```python
from build123d import *

# Parameters (mm, degrees)
F1_DEPTH = 4.6
F2_R     = 1.05
F3_DEPTH = 25


with BuildPart() as f1:
    # F0 (on Top) → F1 (new body)
    with BuildSketch(Plane.XY):
        Polygon((-15.24, 0), (0, 0), (0, 19.245), (-15.24, 19.245), (-15.24, 16.245), (-3, 16.245), (-3, 3), (-15.24, 3), align=None)
    extrude(amount=F1_DEPTH)

    # F2 (on face) → F3 (cut)
    with BuildSketch(Plane.XZ):
        with Locations((-7.62, 2.3)):
            Circle(F2_R)
    extrude(amount=-F3_DEPTH, mode=Mode.SUBTRACT)


solid = f1.part
```
Verification items for the finished model (mm, model axes). A direction names the side the tool comes from. Coordinates: 2 decimals unless noted, no trailing zeros. Loops run counter-clockwise (first coordinate to the right, second up) from the corner with the lowest first, then second, coordinate; pieces in that order, holes last. Notation, with made-up numbers: (80.5, -32) - (126.5, -32) arc R17 ccw to (126.5, -4) - close; hole circle Ø1 at (42.5, -35.75). An arc over 180 degrees is marked (long way). Return JSON: item names as keys, results as strings.
1. Section check C-C, the plane x = -7.62. Record the boundary of the cut face in (y, z) (3 decimals), then the cut area to 3 significant figures.
Established:
{"outline": "(0, 0) - (3, 0) - (3, 1.25) - (0, 1.25) - close; (0, 3.35) - (3, 3.35) - (3, 4.6) - (0, 4.6) - close; (16.245, 0) - (19.245, 0) - (19.245, 1.25) - (16.245, 1.25) - close; (16.245, 3.35) - (19.245, 3.35) - (19.245, 4.6) - (16.245, 4.6) - close", "area": "15.0 mm2"}
2. Mould release check, pull along X, two halves, no side actions. Record for faces 1 (the cylindrical face through (-8.45, 17.72, 1.66)), 2 (the flat face through (-15.24, 18, 2)), 3 (the flat face through (-2.6, 9.8, 0)): +X half, -X half, draft (parallel to the pull), parting line (faces both ways), or undercut.
Established:
{"face 1": "undercut", "face 2": "-X half", "face 3": "draft"}
3. Section check A-A, the plane x = -10.25. Record the boundary of the cut face in (y, z) (3 decimals), then the cut area to 3 significant figures.
Established:
{"outline": "(0, 0) - (3, 0) - (3, 4.6) - (0, 4.6) - close; (16.245, 0) - (19.245, 0) - (19.245, 4.6) - (16.245, 4.6) - close", "area": "27.6 mm2"}
4. Section check B-B, the plane z = 2.3. Record the boundary of the cut face in (x, y) (3 decimals).
Established:
{"outline": "(-15.24, 0) - (-8.67, 0) - (-8.67, 3) - (-15.24, 3) - close; (-15.24, 16.245) - (-8.67, 16.245) - (-8.67, 19.245) - (-15.24, 19.245) - close; (-6.57, 0) - (0, 0) - (0, 19.245) - (-6.57, 19.245) - (-6.57, 16.245) - (-3, 16.245) - (-3, 3) - (-6.57, 3) - close"}
5. Go/stop test with a flat-tipped pin: pin 1 (1 mm diameter, centred on y = 4.5, z = 3, fed in from -X). Record where the tip stops, or that it passes through.
Established:
{"pin 1": "stops at x = -3"}
6. Section check D-D, the plane y = 16.5. Record the boundary of the cut face in (x, z).
Established:
{"outline": "(-15.24, 0) - (0, 0) - (0, 4.6) - (-15.24, 4.6) - close; hole circle Ø2.1 at (-7.62, 2.3)"}
7. Tool access check on faces 4 (the flat face through (-9, 16.245, 2)), 5 (the flat face through (-15.24, 2, 2)). Record the directions out of +Z, -Z, +X, -X, +Y, -Y that give a thin tool (end or side, any length) a straight path to the whole face; none if there is none.
Established:
{"face 4": "+Z, -Z, -X", "face 5": "+Z, -Z, -X, +Y, -Y"}
8. Thickness scan on L1, parallel to Y at x = -9.75, z = 2.4 (3 decimals); L2, parallel to Z at x = -7.62, y = 2.2; L3, parallel to X at y = 8.5, z = 3.3. Record the ranges inside material, lowest first.
Established:
{"L1": "y = 0 to 3, 16.245 to 19.245", "L2": "z = 0 to 1.25, 3.35 to 4.6", "L3": "x = -3 to 0"}
